```python
from build123d import *

# Parameters (mm, degrees)
F0_R        = 18
F0_R_2      = 3.5
F1_DEPTH    = 3
F0_R_3      = 1.5
F2_DEPTH    = 7.5
F2_FACE_R   = 3.5
F2_FACE_R_2 = 1.5
F3_DEPTH    = 12
F5_DEPTH    = 250
F6_R        = 2.51997
F7_DEPTH    = 1


with BuildPart() as f1:
    # F0 (on Front) → F1 (new body)
    with BuildSketch(Plane.XZ):
        Circle(F0_R)
        Circle(F0_R_2, mode=Mode.SUBTRACT)
    extrude(amount=F1_DEPTH)

    # F0 (on Front) → F2 (join)
    with BuildSketch(Plane.XZ):
        Circle(F0_R_2)
        Circle(F0_R_3, mode=Mode.SUBTRACT)
    extrude(amount=F2_DEPTH)

    # F2_face (on face) → F3 (join)
    with BuildSketch(Plane.XZ.offset(7.5)):
        Circle(F2_FACE_R)
        Circle(F2_FACE_R_2, mode=Mode.SUBTRACT)
    extrude(amount=-F3_DEPTH)

    # F4 (on face) → F5 (cut)
    with BuildSketch(Plane.XZ.offset(3)):
        with BuildLine():
            Line((-14.748239, 3), (-3, 3))
            Line((-3, 3), (-3, 14.748239))
            ThreePointArc((-3, 14.748239), (-10.518561, 10.518561), (-14.748239, 3))
        make_face()
        with BuildLine():
            Line((3, 14.748239), (3, 3))
            Line((3, 3), (14.748239, 3))
            ThreePointArc((14.748239, 3), (10.518561, 10.518561), (3, 14.748239))
        make_face()
        with BuildLine():
            Line((-3, -15), (-3, -3))
            Line((-3, -3), (-14.748239, -3))
            ThreePointArc((-14.748239, -3), (-10.575033, -10.665228), (-3, -15))
        make_face()
        with BuildLine():
            Line((14.748239, -3), (3, -3))
            Line((3, -3), (3, -15))
            ThreePointArc((3, -15), (10.575033, -10.665228), (14.748239, -3))
        make_face()
    extrude(amount=-F5_DEPTH, mode=Mode.SUBTRACT)

    # F6 (on face) → F7 (join)
    with BuildSketch(Plane.XZ.offset(7.5)):
        Circle(F6_R)
    extrude(amount=-F7_DEPTH)


solid = f1.part
```
Check sheet for the modelled part. Datum: model origin and axes. Units: mm. A direction names the side the tool comes from. Coordinates: 2 decimals unless noted, no trailing zeros. Order: outer loops, then holes, each group sorted by start corner. A loop starts at its lowest first (then second) coordinate and runs counter-clockwise, first axis right, second up. Notation, with made-up numbers: M 72,52 L 102,52 A26 ccw 102,66 Z; hole C 16,65.25 d2. An arc over 180 degrees is marked long. Write each question's results on one line, items separated by ' | '. Start each with the question number.
1. Cross-section at B-B on x = -6. Record the cut outline in (y, z), and give its area (3 significant figures).
2. Go/stop test with flat-tipped pins: P1, Ø3.5, axis at x = 7, y = -1, coming from the -Z side; P2, Ø1, axis at y = 0, z = 14, coming from the +X side; P3, Ø2.5, axis at x = -10.5, y = -1.5, coming from the -Z side. Record where each tip stops, or that it passes through.
3. Cross-section at A-A on y = -1.25. Record the cut outline in (x, z).
4. Cross-section at C-C on z = 4. Record the cut outline in (x, y).
5. Material ranges on probe 1 along Z at (x, y) = (0, -2.75); probe 2 along Z at (x, y) = (0, 2); probe 3 along X at (y, z) = (-1, 8), recorded low to high.
6. Mould release check, pull along Z, two halves, no side actions. Record for faces 1 (the face through (3.233, -5.219, -1.341)), 2 (the face through (-1.5, -1.08, 0.07)), 3 (the face through (0, -7.5, 0)): +Z half, -Z half, draft (parallel to the pull), parting line (faces both ways), or undercut.
7. Access from +Z, -Z, +X, -X, +Y, -Y to the whole of each face (thin tool, end or side, straight path). Record for faces 4 (the face through (4, -3, 0)), 5 (the face through (0, -6.5, 0)), 6 (the face through (3, -2, -9)), 7 (the face through (0, 4.5, -2)).
8. Cross-section at D-D on z = 0. Record the cut outline in (x, y), and give its area (3 significant figures).
Checks:
1) outline: M -3,-16.97 L 0,-16.97 L 0,-13.93 L -3,-13.93 Z; M -3,-3 L 0,-3 L 0,3 L -3,3 Z; M -3,13.69 L 0,13.69 L 0,16.97 L -3,16.97 Z | area: 37.0 mm²
2) P1: stops at z = -17.22 | P2: stops at x = 11.91 | P3: stops at z = -15.44
3) outline: C 0,0 d36; hole M -14.75,-3 A16 ccw -3,-15 L -3,-3 Z; hole M -14.75,3 L -3,3 L -3,14.75 A16 ccw Z; hole C 0,0 d3; hole M 3,-15 A16 ccw 14.75,-3 L 3,-3 Z; hole M 3,3 L 14.75,3 A16 ccw 3,14.75 Z
4) outline: M -17.55,-3 L -14.47,-3 L -14.47,0 L -17.55,0 Z; M -3,-3 L 3,-3 L 3,0 L -3,0 Z; M 14.47,-3 L 17.55,-3 L 17.55,0 L 14.47,0 Z
5) probe 1: z = -18 to -1.5, 1.5 to 18 | probe 2: z = -3.5 to -1.5, 1.5 to 3.5 | probe 3: x = -16.12 to -12.57, -3 to 3, 12.57 to 16.12
6) face 1: parting line | face 2: undercut | face 3: draft
7) face 4: -Y | face 5: +Y | face 6: +Y, -Y | face 7: +Z, -Z, +X, -X, +Y
8) outline: M -18,-3 L -3.5,-3 L -3.5,-7.5 L 3.5,-7.5 L 3.5,-3 L 18,-3 L 18,0 L 3.5,0 L 3.5,4.5 L 1.5,4.5 L 1.5,-6.5 L -1.5,-6.5 L -1.5,4.5 L -3.5,4.5 L -3.5,0 L -18,0 Z | area: 138 mm²
